Check sheet for the modelled part. Datum: model origin and axes. Units: mm. Face numbers are marked on the shaded views. Round coordinates to 2 decimals unless told otherwise and drop trailing zeros. Write each loop counter-clockwise with the first axis right and the second up, starting at its lowest first coordinate (ties: lowest second). Pieces come first, ordered by that corner, then holes.
Item 1: Material ranges on line 1 (Z direction, x = 33.5, y = 5.75); line 2 (X direction, y = 4.5, z = -14.5); line 3 (X direction, y = 4, z = 0.5), recorded low to high.
Item 2: Release check for a two-part mould opening along X. For the marked faces 1 and 2 record: +X half, -X half, draft (parallel to the pull), parting line (faces both ways), or undercut.
Item 3: Cross-section at B-B on z = -20. Enter the section's corners in (x, y), plus the area to 3 significant figures.
Item 4: Cross-section at A-A on z = 9. Enter the section's corners in (x, y).
Item 5: Go/stop test with flat-tipped pins: pin 1 Ø3 at (y, z) = (3.5, -37) entering from -X; pin 2 Ø1.9 at (x, y) = (37.5, 3) entering from -Z (3 decimals); pin 3 Ø1.5 at (y, z) = (5.5, -25.5) entering from -X. Record where each tip stops, or that it passes through.
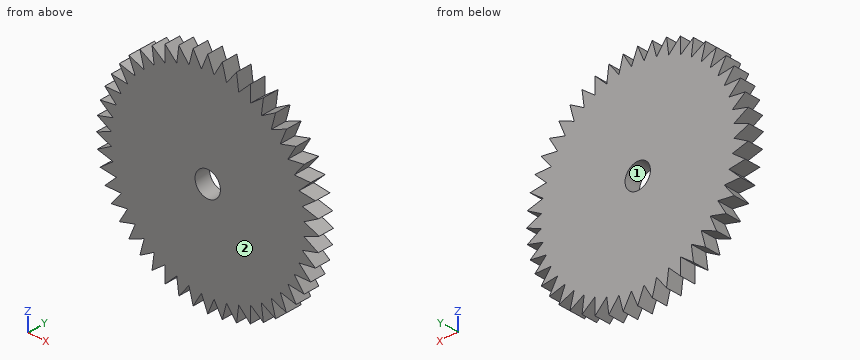
from build123d import *

# Parameters (mm, degrees)
BOSS_EXTRUDE1_DEPTH = 6.35
SKETCH3_R           = 5.08
CUT_EXTRUDE3_DEPTH  = 6.35


with BuildPart() as part:
    # Sketch2 → Boss-Extrude1 (new body)
    with BuildSketch(Plane(origin=(0, 0, 0), x_dir=(1, 0, 0), z_dir=(0, 1, 0))):
        Polygon((-17.07562385, 34.625939831), (-17.07562385, 41.224202684), (-12.409947442, 36.558526277), (-11.548701317, 43.100340077), (-7.531933394, 37.865586202), (-5.824177303, 44.2390187), (-2.525045876, 38.524755449), (0, 44.620755449), (2.525045876, 38.524755449), (5.824177303, 44.2390187), (7.531933394, 37.865586202), (11.548701317, 43.100340077), (12.409947442, 36.558526277), (17.07562385, 41.224202684), (17.07562385, 34.625939831), (22.310377724, 38.642707755), (21.449131599, 32.100893955), (27.16339485, 35.400025382), (25.45563876, 29.026592883), (31.55163876, 31.55163876), (29.026592883, 25.45563876), (35.400025382, 27.163394851), (32.100893955, 21.449131599), (38.642707755, 22.310377724), (34.625939831, 17.07562385), (41.224202684, 17.07562385), (36.558526277, 12.409947443), (43.100340077, 11.548701317), (37.865586202, 7.531933394), (44.2390187, 5.824177303), (38.524755449, 2.525045876), (44.620755449, 0), (38.524755449, -2.525045876), (44.2390187, -5.824177303), (37.865586202, -7.531933394), (43.100340077, -11.548701317), (36.558526277, -12.409947442), (41.224202684, -17.07562385), (34.625939831, -17.07562385), (38.642707755, -22.310377724), (32.100893955, -21.449131599), (35.400025382, -27.16339485), (29.026592883, -25.45563876), (31.55163876, -31.55163876), (25.45563876, -29.026592883), (27.163394851, -35.400025382), (21.449131599, -32.100893955), (22.310377724, -38.642707755), (17.07562385, -34.625939831), (17.07562385, -41.224202684), (12.409947443, -36.558526277), (11.548701317, -43.100340077), (7.531933394, -37.865586202), (5.824177303, -44.2390187), (2.525045876, -38.524755449), (0, -44.620755449), (-2.525045876, -38.524755449), (-5.824177303, -44.2390187), (-7.531933394, -37.865586202), (-11.548701317, -43.100340077), (-12.409947442, -36.558526277), (-17.07562385, -41.224202684), (-17.07562385, -34.625939831), (-22.310377724, -38.642707755), (-21.449131599, -32.100893955), (-27.16339485, -35.400025382), (-25.455638759, -29.026592883), (-31.551638759, -31.55163876), (-29.026592883, -25.45563876), (-35.400025382, -27.16339485), (-32.100893955, -21.449131599), (-38.642707755, -22.310377724), (-34.625939831, -17.07562385), (-41.224202684, -17.07562385), (-36.558526277, -12.409947442), (-43.100340077, -11.548701317), (-37.865586202, -7.531933394), (-44.2390187, -5.824177303), (-38.524755449, -2.525045876), (-44.620755449, 0), (-38.524755449, 2.525045876), (-44.2390187, 5.824177303), (-37.865586202, 7.531933394), (-43.100340077, 11.548701317), (-36.558526277, 12.409947442), (-41.224202684, 17.07562385), (-34.625939831, 17.07562385), (-38.642707755, 22.310377724), (-32.100893955, 21.449131599), (-35.400025382, 27.16339485), (-29.026592883, 25.45563876), (-31.55163876, 31.55163876), (-25.45563876, 29.026592883), (-27.16339485, 35.400025382), (-21.449131599, 32.100893955), (-22.310377724, 38.642707755), align=None)
    extrude(amount=BOSS_EXTRUDE1_DEPTH)

    # Sketch3 → Cut-Extrude3 (cut)
    with BuildSketch(Plane(origin=(0, 6.35, 0), x_dir=(1, 0, 0), z_dir=(0, 1, 0))):
        with Locations(Location((0, 0, 0), (0, 0, 270))):
            Circle(SKETCH3_R)
    extrude(amount=-CUT_EXTRUDE3_DEPTH, mode=Mode.SUBTRACT)


solid = part.part
Response values:
1. line 1: z = -26.65 to -23.87, -21.63 to 21.63, 23.87 to 26.65
1. line 2: x = -38.65 to 38.65
1. line 3: x = -43.41 to -5.06, 5.06 to 43.41
2. face 1: undercut
2. face 2: draft
3. outline: (-36.87, 0) - (36.87, 0) - (36.87, 6.35) - (-36.87, 6.35) - close
3. area: 468 mm2
4. outline: (-39.78, 0) - (39.78, 0) - (39.78, 6.35) - (-39.78, 6.35) - close
5. pin 1: stops at x = -22.29
5. pin 2: stops at z = -22.285
5. pin 3: stops at x = -34.87
